The listing builds one solid part. Answer for the finished solid, in the listing's coordinates (mm). Face numbers are marked on the shaded views. A direction names the side the tool comes from. Give positions to 0.01 mm unless a question says otherwise; leave off trailing zeros. Write each loop counter-clockwise with the first axis right and the second up, starting at its lowest first coordinate (ties: lowest second). Pieces come first, ordered by that corner, then holes. Notation, with made-up numbers: (71.5, 14) - (79.5, 14) arc R30 cw to (79.5, 46) - close; hole circle Ø5 at (-3, 70). An arc over 180 degrees is marked (long way). Use a Markdown table: item, result. Add a question column.
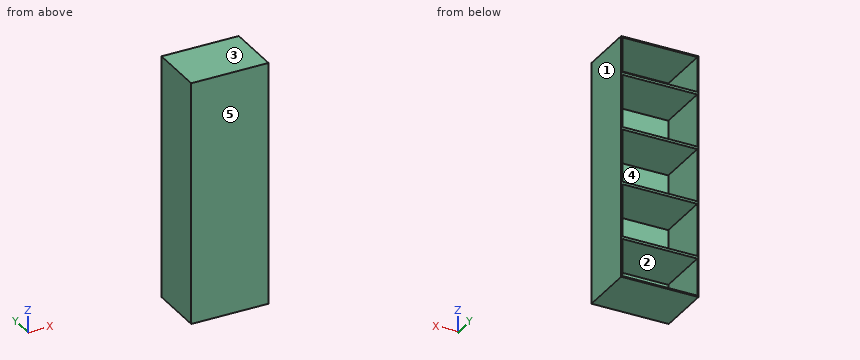
from build123d import *

# Parameters (mm, degrees)
CROQUIS1_W              = 700
CROQUIS1_H              = 500
SALIENTE_EXTRUIR1_DEPTH = 2200
VACIADO1_T              = -10
CROQUIS2_W              = 680
CROQUIS2_H              = 23.319411046
SALIENTE_EXTRUIR2_DEPTH = 488
MATRIZL1_COUNT          = 4
MATRIZL1_PITCH          = 500


with BuildPart() as part:
    # Croquis1 → Saliente-Extruir1 (new body)
    with BuildSketch(Plane.XY):
        Rectangle(CROQUIS1_W, CROQUIS1_H)
    extrude(amount=SALIENTE_EXTRUIR1_DEPTH)

    # Vaciado1
    vaciado1_openings = [part.faces().sort_by_distance(p)[0] for p in [
        (0, 250, 1100),
    ]]
    offset(amount=VACIADO1_T, openings=vaciado1_openings, kind=Kind.INTERSECTION)

    # Croquis2 → Saliente-Extruir2 (add)
    with BuildSketch(Plane(origin=(0, -240, 0), x_dir=(1, 0, 0), z_dir=(0, 1, 0))):
        with Locations((0, -361.692736208)):
            Rectangle(CROQUIS2_W, CROQUIS2_H)
    saliente_extruir2 = extrude(amount=SALIENTE_EXTRUIR2_DEPTH)

    # MatrizL1: Saliente-Extruir2 ×4
    with Locations(*[(0, 0, i * MATRIZL1_PITCH) for i in range(1, MATRIZL1_COUNT)]):
        add(saliente_extruir2)


solid = part.part
1. Given P1, Ø8, axis at x = 277.5, z = 1422.5, coming from the +Y side; P2, Ø7, axis at x = 110, z = 1863, coming from the +Y side, each flat-ended and moving along its own axis, determine where each tip first touches the part or whether it passes through.
2. Which of the six approach directions +Z, -Z, +X, -X, +Y, -Y give full straight-line access (tool end or side, diameter ignored) to the marked faces 4 and 5?
3. The part is cut by section A-A (y = -42.5). Give the vertices of the cut face in (x, z), and give its area (3 significant figures).
4. The part is cut by section B-B (z = 272). Give the vertices of the cut face in (x, y), and give its area (3 significant figures).
5. For a pull along X with two mould halves and no side action, classify the marked faces 1, 2 and 3 as released by +X, released by -X, zero draft, split by the parting line, or undercut.
6. The part is cut by section C-C (x = -229). Give the vertices of the cut face in (y, z), and give its area (3 significant figures).
7. Consider L1, parallel to Z at x = -313.5, y = -68.5; L2, parallel to X at y = -122.5, z = 403; L3, parallel to Y at x = 51, z = 1027. Determine where each line is inside the solid, lowest interval first. Write a range as [from, to].
Check values:
| question | item | result |
|---|---|---|
| 1 | P1 | stops at y = -240 |
| 1 | P2 | stops at y = 248 |
| 2 | face 4 | +Y |
| 2 | face 5 | +Z, -Z, +X, -X, -Y |
| 3 | outline | (-350, 0) - (350, 0) - (350, 2200) - (-350, 2200) - close; hole (-340, 10) - (340, 10) - (340, 350.03) - (-340, 350.03) - close; hole (-340, 373.35) - (340, 373.35) - (340, 850.03) - (-340, 850.03) - close; hole (-340, 873.35) - (340, 873.35) - (340, 1350.03) - (-340, 1350.03) - close; hole (-340, 1373.35) - (340, 1373.35) - (340, 1850.03) - (-340, 1850.03) - close; hole (-340, 1873.35) - (340, 1873.35) - (340, 2190) - (-340, 2190) - close |
| 3 | area | 121,000 mm2 |
| 4 | outline | (-350, -250) - (350, -250) - (350, 250) - (340, 250) - (340, -240) - (-340, -240) - (-340, 250) - (-350, 250) - close |
| 4 | area | 16,800 mm2 |
| 5 | face 1 | released by +X |
| 5 | face 2 | undercut |
| 5 | face 3 | zero draft |
| 6 | outline | (-250, 0) - (250, 0) - (250, 10) - (-240, 10) - (-240, 350.03) - (248, 350.03) - (248, 373.35) - (-240, 373.35) - (-240, 850.03) - (248, 850.03) - (248, 873.35) - (-240, 873.35) - (-240, 1350.03) - (248, 1350.03) - (248, 1373.35) - (-240, 1373.35) - (-240, 1850.03) - (248, 1850.03) - (248, 1873.35) - (-240, 1873.35) - (-240, 2190) - (250, 2190) - (250, 2200) - (-250, 2200) - close |
| 6 | area | 77,300 mm2 |
| 7 | L1 | z = [0, 10], [350.03, 373.35], [850.03, 873.35], [1350.03, 1373.35], [1850.03, 1873.35], [2190, 2200] |
| 7 | L2 | x = [-350, -340], [340, 350] |
| 7 | L3 | y = [-250, -240] |
